Work out the finished part from the listing and answer in its coordinate system (mm). A direction names the side the tool comes from. Coordinates: 2 decimals unless noted, no trailing zeros. Write each loop counter-clockwise with the first axis right and the second up, starting at its lowest first coordinate (ties: lowest second). Pieces come first, ordered by that corner, then holes. Notation, with made-up numbers: M -6.5,22 L 26.5,22 A17 cw 26.5,50 Z; hole C 3,34 d8. An arc over 180 degrees is marked long. Answer as CSV lines item,"result". Start each with the question number.
(1) A cutting plane is placed at C-C on x = 22. Give the vertices of the cut face in (y, z), then the cut area to 3 significant figures.
(2) Flat-ended cylindrical pins translate along their axes: P1, Ø3, axis at y = 0, z = 11.5, coming from the +X side; P2, Ø2, axis at x = 25.5, z = 13, coming from the +Y side; P3, Ø1.4, axis at y = 0.5, z = 12.5, coming from the -X side; P4, Ø2, axis at x = -21.5, z = 7, coming from the +Y side. Find the tip coordinate at first contact, or state that the pin passes through.
(3) A cutting plane is placed at B-B on y = 0.5. Give the vertices of the cut face in (x, z), then the cut area to 3 significant figures.
(4) Find the intervals of material crossed by L1, parallel to X at y = -1, z = 5.5; L2, parallel to Z at x = -14.5, y = 4; L3, parallel to Y at x = -29, z = 8.25, in increasing order. Write a range as [from, to].
(5) A cutting plane is placed at D-D on y = -4. Give the vertices of the cut face in (x, z).
(6) For faces 1 (the flat face through (-27, -2.4, 10)), 2 (the cylindrical face through (25.38, 2, 5.14)), 3 (the flat face through (27, 2.4, 10)), 4 (the flat face through (-25, 0, 10)), determine the directions among +Z, -Z, +X, -X, +Y, -Y from which every point of the face is accessible in a straight line to the end or side of a thin tool.
(7) A cutting plane is placed at A-A on z = 6.25. Give the vertices of the cut face in (x, y).
(8) The mould has two halves that part along X. Classify faces 5 (the flat face through (0, 0, 5)), 6 (the flat face through (-29.8, 0, 10)), 7 (the flat face through (29.8, 0, 10)), 8 (the flat face through (27, 0, 15)): released by +X, released by -X, zero draft, split by the parting line, or undercut.
Autodesk Inventor part; units mm, degrees
ref_plane "YZ Plane" through (0, 0, 0) normal (1, 0, 0) x (0, 1, 0)
ref_plane "XZ Plane" through (0, 0, 0) normal (0, 1, 0) x (-1, 0, 0)
ref_plane "XY Plane" through (0, 0, 0) normal (0, 0, 1) x (1, 0, 0)
sketch "Sketch1" plane through (0, 0, 0) normal (0, 0, 1) x (1, 0, 0)
  line L0 (-35, 5) -> (35, 5)
  line L1 (35, 5) -> (35, -5)
  line L2 (35, -5) -> (-35, -5)
  line L3 (-35, -5) -> (-35, 5)
  line L4 (-35, 5) -> (35, -5) construction
  line L5 (35, 5) -> (-35, -5) construction
  point P0 (0, 0)
  dimension "d0" = 70
  dimension "d1" = 10
extrude "Extrusion1" add sketch "Sketch1" along normal blind 5
sketch "Sketch2" plane through (0, 0, 5) normal (0, 0, 1) x (1, 0, 0)
  line L0 (-29.8, 2.4) -> (-25, 2.4)
  line L1 (-25, 2.4) -> (-25, -2.4)
  line L2 (-25, -2.4) -> (-29.8, -2.4)
  line L3 (-29.8, -2.4) -> (-29.8, 2.4)
  line L4 (-29.8, 2.4) -> (-25, -2.4) construction
  line L5 (-25, 2.4) -> (-29.8, -2.4) construction
  line L6 (35, 5) -> (-35, 5) construction
  line L7 (-35, -5) -> (35, -5) construction
  line L8 (0, 5) -> (0, -5) construction
  line L9 (29.8, 2.4) -> (25, 2.4)
  line L10 (25, 2.4) -> (25, -2.4)
  line L11 (25, -2.4) -> (29.8, -2.4)
  line L12 (29.8, -2.4) -> (29.8, 2.4)
  point P0 (0, 0)
  point P1 (-27.4, 0)
  point P2 (-25, 0)
  dimension "d4" = 4.8
  dimension "d5" = 4.8
  dimension "d6" = 25
extrude "Extrusion2" add sketch "Sketch2" along normal blind 10
chamfer "Chamfer1" distance 1 angle 45 8 edges at (-29.8, 2.4, 10) (-25, 2.4, 10) (-29.8, -2.4, 10) (-25, -2.4, 10) (25, 2.4, 10) (29.8, 2.4, 10) (29.8, -2.4, 10) (25, -2.4, 10)
fillet "Fillet1" radius 0.5 8 edges at (-27.4, 2.4, 5) (-25.5, 1.9, 5) (-25, 0, 5) (-25.5, -1.9, 5) (-27.4, -2.4, 5) (-29.3, -1.9, 5) (-29.8, 0, 5) (-29.3, 1.9, 5)
fillet "Fillet2" radius 0.5 8 edges at (25, 0, 5) (25.5, 1.9, 5) (27.4, 2.4, 5) (29.3, 1.9, 5) (29.8, 0, 5) (29.3, -1.9, 5) (27.4, -2.4, 5) (25.5, -1.9, 5)
properties part number "UNION_INTERNA"
Here are the results:
1,outline,"M -5,0 L 5,0 L 5,5 L -5,5 Z"
1,area,"50.0 mm^2"
2,P1,"stops at x = 29.8"
2,P2,"stops at y = 2.4"
2,P3,"stops at x = -29.8"
2,P4,"passes through"
3,outline,"M -35,0 L 35,0 L 35,5 L 30.3,5 A0.5 cw 29.8,5.5 L 29.8,15 L 25,15 L 25,5.5 A0.5 cw 24.5,5 L -24.5,5 A0.5 cw -25,5.5 L -25,15 L -29.8,15 L -29.8,5.5 A0.5 cw -30.3,5 L -35,5 Z"
3,area,"446 mm^2"
4,L1,"x = [-29.8, -25], [25, 29.8]"
4,L2,"z = [0, 5]"
4,L3,"y = [-2.2, 2.2]"
5,outline,"M -35,0 L 35,0 L 35,5 L -35,5 Z"
6,face 1,"+Z, +X, -X, -Y"
6,face 2,"+Z, +Y"
6,face 3,"+Z, +X, -X, +Y"
6,face 4,"+Z, +Y, -Y"
7,outline,"M -29.8,-1.4 L -28.8,-2.4 L -26,-2.4 L -25,-1.4 L -25,1.4 L -26,2.4 L -28.8,2.4 L -29.8,1.4 Z; M 25,-1.4 L 26,-2.4 L 28.8,-2.4 L 29.8,-1.4 L 29.8,1.4 L 28.8,2.4 L 26,2.4 L 25,1.4 Z"
8,face 5,"undercut"
8,face 6,"released by -X"
8,face 7,"released by +X"
8,face 8,"zero draft"
